Verification items for this drawing (mm, ordinates from the low corner). A direction names the side the tool comes from. Coordinates: 2 decimals unless noted, no trailing zeros. Order: outer loops, then holes, each group sorted by start corner. A loop starts at its lowest first (then second) coordinate and runs counter-clockwise, first axis right, second up. Notation, with made-up numbers: M 75,22 L 125,22 A33 cw 125,61 Z; hole C -27,-20.5 d11. An arc over 180 degrees is marked long. One line per item, written item: value. Start each with the question number.
1) Sectioned sample at C-C, the plane x = 9.25. Enter the section's corners in (y, z), then the cut area to 3 significant figures.
2) Thickness scan on L1, parallel to Z at x = 1, y = 10; L2, parallel to Y at x = 3.25, z = 16; L3, parallel to Z at x = 4.75, y = 45. Record the ranges inside material, lowest first. Write a range as from..to.
3) Go/stop test with flat-tipped pins: P1, Ø5, axis at x = 14, z = 42, coming from the -Y side; P2, Ø1.5, axis at x = 2, y = 32, coming from the +Z side; P3, Ø5, axis at y = 10, z = 60, coming from the -X side; P4, Ø1, axis at x = 4, z = 23, coming from the +Y side. Record where each tip stops, or that it passes through.
4) Access from +Z, -Z, +X, -X, +Y, -Y to the whole of each face (thin tool, end or side, straight path). Record for the marked faces 1 and 2.
5) Sectioned sample at D-D, the plane z = 31. Enter the section's corners in (x, y).
6) Sectioned sample at A-A, the plane z = 23. Enter the section's corners in (x, y), then the cut area to 3 significant figures.
7) Sectioned sample at B-B, the plane y = 10. Enter the section's corners in (x, z).
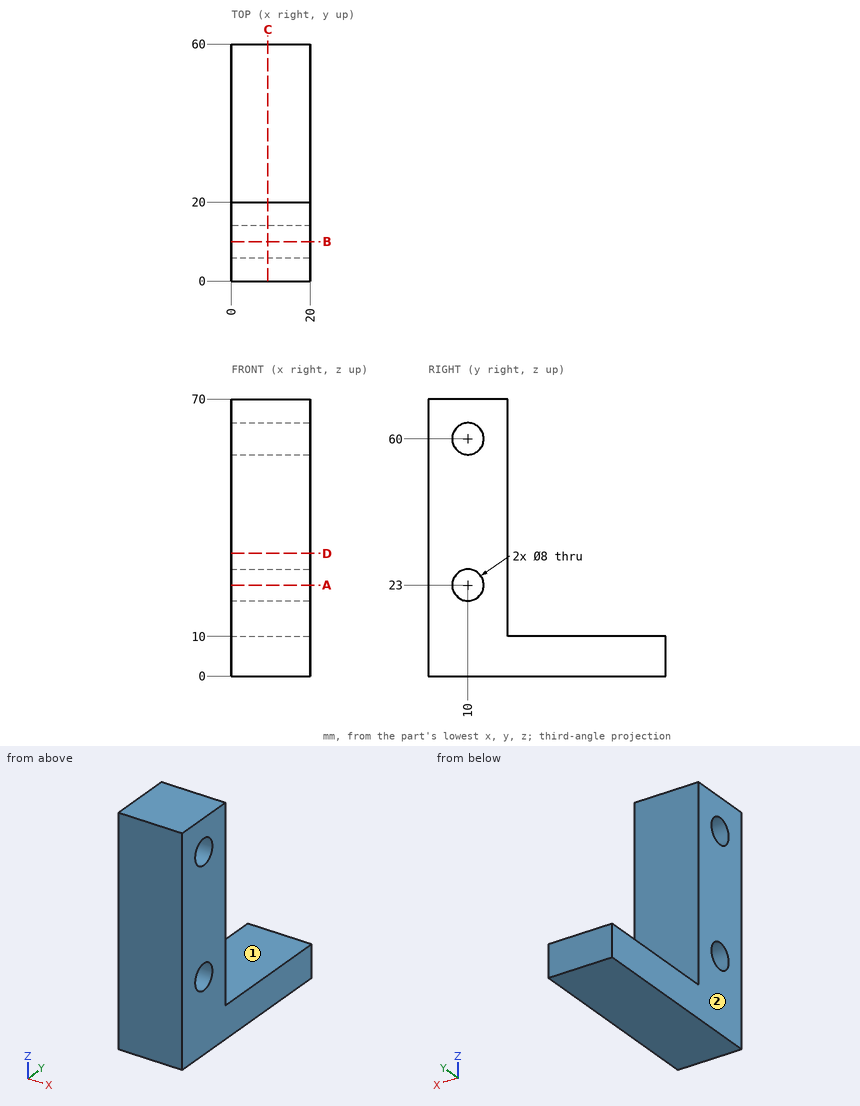
Final values:
1. outline: M 0,0 L 60,0 L 60,10 L 20,10 L 20,70 L 0,70 Z; hole C 10,23 d8; hole C 10,60 d8
1. area: 1,700 mm^2
2. L1: z = 0..19, 27..56, 64..70
2. L2: y = 0..20
2. L3: z = 0..10
3. P1: stops at y = 0
3. P2: stops at z = 10
3. P3: passes through
3. P4: stops at y = 20
4. face 1: +Z, +X, -X, +Y
4. face 2: +Z, -Z, -X, +Y, -Y
5. outline: M 0,0 L 20,0 L 20,20 L 0,20 Z
6. outline: M 0,0 L 20,0 L 20,6 L 0,6 Z; M 0,14 L 20,14 L 20,20 L 0,20 Z
6. area: 240 mm^2
7. outline: M 0,0 L 20,0 L 20,19 L 0,19 Z; M 0,27 L 20,27 L 20,56 L 0,56 Z; M 0,64 L 20,64 L 20,70 L 0,70 Z
